The model under review builds one solid part; all positions refer to its coordinate system, in mm. Give positions to 0.01 mm unless a question says otherwise; leave off trailing zeros. Loops run counter-clockwise (first coordinate to the right, second up) from the corner with the lowest first, then second, coordinate; pieces in that order, holes last. Notation, with made-up numbers: M 33.25,51.5 L 74.25,51.5 A14 ccw 74.25,70.5 Z; hole C 35.5,47 d9. An arc over 180 degrees is marked long. Return JSON: item names as keys, results as strings.
```python
from build123d import *

# Parameters (mm, degrees)
SKETCH1_R               = 1.1
BOSS_EXTRUDE1_DEPTH     = 1
SKETCH3_R               = 12.7
CUT_EXTRUDE1_DEPTH      = 2.979898987
CUT_EXTRUDE1_DEPTH_BACK = 2.272792206
CUT_EXTRUDE2_REACH      = 3
SKETCH4_R               = 9.430256121


with BuildPart() as part:
    # Sketch1 → Boss-Extrude1 (new body)
    with BuildSketch(Plane(origin=(0, 0, 0), x_dir=(1, 0, 0), z_dir=(0, 1, 0))):
        with BuildLine():
            Line((-1.8, -13.375), (-1.8, 13.375))
            ThreePointArc((-1.8, 13.375), (0, 15.175), (1.8, 13.375))
            Line((1.8, 13.375), (1.8, -13.375))
            ThreePointArc((1.8, -13.375), (0, -15.175), (-1.8, -13.375))
        make_face()
        with Locations((0, -13.75)):
            Circle(SKETCH1_R, mode=Mode.SUBTRACT)
        with Locations((0, 13.75)):
            Circle(SKETCH1_R, mode=Mode.SUBTRACT)
    extrude(amount=BOSS_EXTRUDE1_DEPTH)

    # Sketch3 → Cut-Extrude1 (cut, two sides)
    with BuildSketch(Plane(origin=(0, 0, 0), x_dir=(0.707106781, -0.707106781, 0), z_dir=(0.707106781, 0.707106781, 0))) as cut_extrude1_sk:
        with Locations((12.7, 0)):
            Circle(SKETCH3_R)
    extrude(amount=CUT_EXTRUDE1_DEPTH, mode=Mode.SUBTRACT)
    extrude(cut_extrude1_sk.sketch, amount=-CUT_EXTRUDE1_DEPTH_BACK, mode=Mode.SUBTRACT)

    # Sketch4 → Cut-Extrude2 (cut, up to next)
    with BuildSketch(Plane.XZ, mode=Mode.PRIVATE) as cut_extrude2_sk1:
        with Locations((9.430256121, 0)):
            Circle(SKETCH4_R)
    cut_extrude2_tool1 = extrude(cut_extrude2_sk1.sketch, amount=-CUT_EXTRUDE2_REACH, mode=Mode.PRIVATE) & part.part
    add(cut_extrude2_tool1.solids().sort_by_distance((9.430256, 0, 0))[0], mode=Mode.SUBTRACT)


solid = part.part
```
1) Consider section D-D on x = -0.45. Write out the cut boundary in (y, z).
From the geometry:
{"outline": "M 0,-15.12 L 1,-15.12 L 1,-14.75 L 0,-14.75 Z; M 0,-12.75 L 1,-12.75 L 1,12.75 L 0,12.75 Z; M 0,14.75 L 1,14.75 L 1,15.12 L 0,15.12 Z"}
2) Consider section A-A on x = 1.45. Write out the cut boundary in (y, z).
From the geometry:
{"outline": "M 0,-14.44 L 1,-14.44 L 1,-5.02 L 0,-5.02 Z; M 0,5.02 L 1,5.02 L 1,14.44 L 0,14.44 Z"}
3) Consider section C-C on z = -13.75. Write out the cut boundary in (x, y).
From the geometry:
{"outline": "M -1.76,0 L -1.1,0 L -1.1,1 L -1.76,1 Z; M 1.1,0 L 1.76,0 L 1.76,1 L 1.1,1 Z"}
4) Consider section B-B on y = 0.25. Write out the cut boundary in (x, z) (3 decimals), then the cut area to 3 significant figures.
From the geometry:
{"outline": "M -1.8,-13.375 A1.8 ccw 1.8,-13.375 L 1.8,-5.542 A9.43 cw 1.8,5.542 L 1.8,13.375 A1.8 ccw -1.8,13.375 Z; hole C 0,-13.75 d2.2; hole C 0,13.75 d2.2", "area": "85.3 mm²"}
5) Wall thickness on L1, parallel to Z at x = -0.5, y = 0.95; L2, parallel to Z at x = -0.3, y = 0.7; L3, parallel to X at y = 0.3, z = -13.75: over which ranges is each line inside the solid? List them lowest first. Write a range as from..to.
From the geometry:
{"L1": "-15.1..-14.73, -12.77..12.77, 14.73..15.1", "L2": "-15.15..-14.81, -12.69..12.69, 14.81..15.15", "L3": "-1.76..-1.1, 1.1..1.76"}
6) The part is to be moulded in two halves that separate along Z. For faces 1 (the face through (0, 0.5, 0.1)), 2 (the face through (-0.238, 0.493, -12.676)), 3 (the face through (-1.8, 0.5, 0.2)), 4 (the face through (-0.04, 0.493, -15.175)), say which applies: released by +Z, released by -Z, zero draft, split by the parting line, or undercut.
From the geometry:
{"face 1": "undercut", "face 2": "undercut", "face 3": "zero draft", "face 4": "released by -Z"}
